The drawing under review shows one solid part. Ordinate dimensions are in mm from its lowest x, y, z. A direction names the side the tool comes from. Give positions to 0.01 mm unless a question says otherwise; leave off trailing zeros. Loops run counter-clockwise (first coordinate to the right, second up) from the corner with the lowest first, then second, coordinate; pieces in that order, holes last.
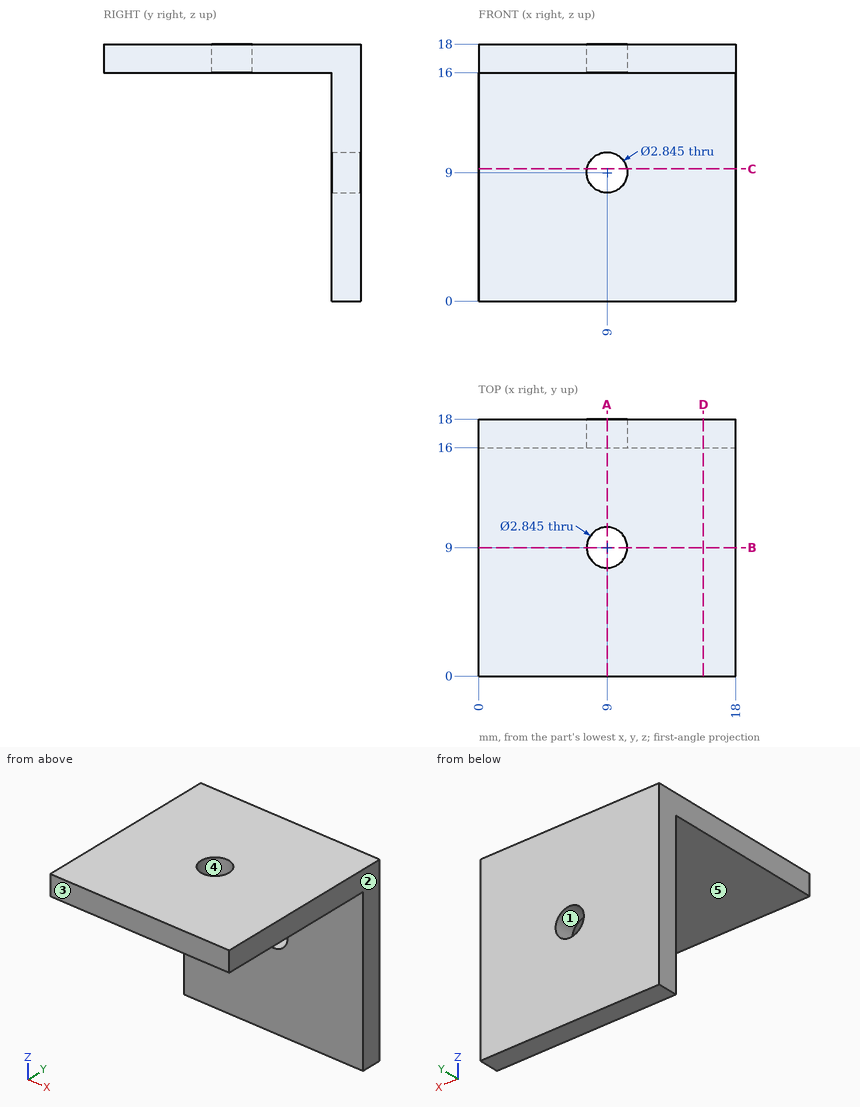
Item 1: Take a section at B-B on y = 9. Give the boundary of the cut face in (x, z).
Answer:
outline: (0, 16) - (7.58, 16) - (7.58, 18) - (0, 18) - close; (10.42, 16) - (18, 16) - (18, 18) - (10.42, 18) - close
Item 2: Take a section at C-C on z = 9.25. Give the boundary of the cut face in (x, y), and give its area (3 significant figures).
Answer:
outline: (0, 16) - (7.6, 16) - (7.6, 18) - (0, 18) - close; (10.4, 16) - (18, 16) - (18, 18) - (10.4, 18) - close
area: 30.4 mm2
Item 3: For L1, parallel to X at y = 16.8, z = 9, list the stretches that pass through material, from the lowest coordinate up.
Answer:
L1: x = 0 to 7.58, 10.42 to 18
Item 4: Take a section at D-D on x = 15.75. Give the boundary of the cut face in (y, z).
Answer:
outline: (0, 16) - (16, 16) - (16, 0) - (18, 0) - (18, 18) - (0, 18) - close
Item 5: The part is to be moulded in two halves that separate along X. For the marked faces 1, 2 and 3, say which applies: released by +X, released by -X, zero draft, split by the parting line, or undercut.
Answer:
face 1: undercut
face 2: released by +X
face 3: zero draft
Item 6: Take a section at A-A on x = 9. Give the boundary of the cut face in (y, z), and give its area (3 significant figures).
Answer:
outline: (0, 16) - (7.58, 16) - (7.58, 18) - (0, 18) - close; (10.42, 16) - (16, 16) - (16, 10.42) - (18, 10.42) - (18, 18) - (10.42, 18) - close; (16, 0) - (18, 0) - (18, 7.58) - (16, 7.58) - close
area: 56.6 mm2
Item 7: Clearance check with flat-ended pins moving along their axes: pin 1 Ø5 at (x, z) = (8, 5) entering from -Y; pin 2 Ø8 at (x, y) = (11.5, 10) entering from -Z; pin 3 Ø2.5 at (x, y) = (9, 9) entering from -Z. State where each tip first meets the part, or that it passes through.
Answer:
pin 1: stops at y = 16
pin 2: stops at z = 16
pin 3: passes through
Item 8: Tool access review of the marked faces 4 and 5: name each direction out of +Z, -Z, +X, -X, +Y, -Y from which nothing blocks a thin tool from reaching the whole face with its end or side.
Answer:
face 4: +Z, -Z
face 5: -Z, +X, -X, -Y
